Geometry check sheet. Reference: drawing and pictorial views, mm from the part's lowest x, y, z. A direction names the side the tool comes from. Give positions to 0.01 mm unless a question says otherwise; leave off trailing zeros. Write each loop counter-clockwise with the first axis right and the second up, starting at its lowest first coordinate (ties: lowest second). Pieces come first, ordered by that corner, then holes. Notation, with made-up numbers: M -13,87.25 L 3,87.25 A14 cw 3,95.25 Z; hole C -3,-12 d5. An arc over 180 degrees is marked long. Write item = value, one per line. Start each with the question number.
1) Cross-section at A-A, the plane z = 5.75. Record the cut outline in (x, y), plus the area to 3 significant figures.
2) Go/stop test with flat-tipped pins: pin 1 (6 mm diameter, centred on x = 31, z = 7.5, fed in from +Y); pin 2 (1.8 mm diameter, centred on y = 18, z = 4.5, fed in from +X); pin 3 (6 mm diameter, centred on y = 27.5, z = 6, fed in from +X). Record where each tip stops, or that it passes through.
3) Scan lines: line 1 along Y through (x, z) = (15, 6); line 2 along Y through (x, z) = (26, 7.75); line 3 along X through (y, z) = (30, 9.25). Record each from-to range of solid material in increasing order. Write a range as [from, to].
4) Cross-section at B-B, the plane x = 16. Record the cut outline in (y, z), plus the area to 3 significant figures.
5) Access from +Z, -Z, +X, -X, +Y, -Y to the whole of each face (thin tool, end or side, straight path). Record for the marked faces 1 and 2.
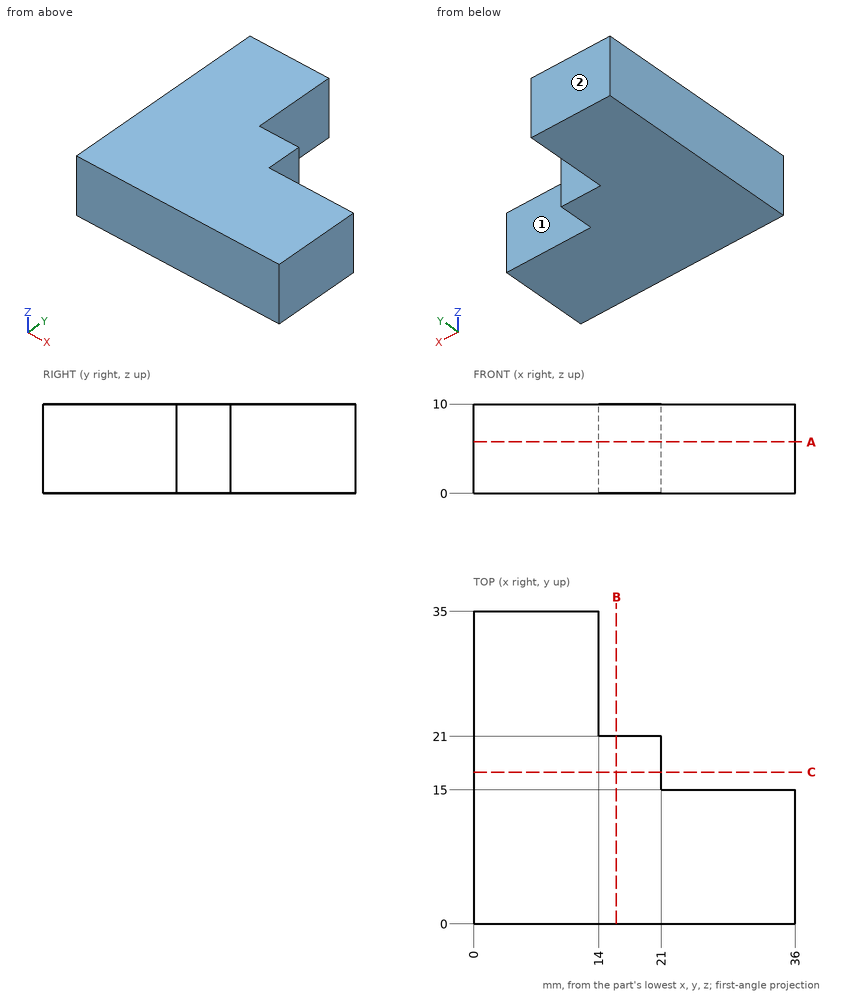
Reply:
q1.outline = M 0,0 L 36,0 L 36,15 L 21,15 L 21,21 L 14,21 L 14,35 L 0,35 Z
q1.area = 862 mm2
q2.pin_1 = 15
q2.pin_2 = 21
q2.pin_3 = 14
q3.line_1 = [0, 21]
q3.line_2 = [0, 15]
q3.line_3 = [0, 14]
q4.outline = M 0,0 L 21,0 L 21,10 L 0,10 Z
q4.area = 210 mm2
q5.face_1 = +Z, -Z, +X, +Y
q5.face_2 = +Z, -Z, +X, -X, +Y
